```python
from build123d import *
from build123d.topology import SkipClean

# Parameters (mm, degrees)
BOSS_EXTRUDE1_DEPTH     = 8
FILLET2_R               = 2
SKETCH3_R               = 2.839661977
CUT_EXTRUDE1_DEPTH      = 8
SKETCH4_R               = 3.5
CUT_EXTRUDE2_DEPTH      = 8
CUT_EXTRUDE3_DEPTH      = 2.5
CUT_EXTRUDE3_DEPTH_BACK = 2.5
SKETCH5_R               = 32.5
SKETCH6_W               = 4.5
SKETCH6_H               = 19
CUT_EXTRUDE4_DEPTH      = 10
SKETCH7_R               = 1.75
CUT_EXTRUDE5_DEPTH      = 51
FILLET3_START           = -1
FILLET3_DEPTH           = 10
FILLET4_START           = -1
FILLET4_DEPTH           = 10
SKETCH9_W               = 5
SKETCH9_H               = 5
CUT_EXTRUDE6_DEPTH      = 51
SKETCH10_R              = 1.75
CUT_EXTRUDE7_DEPTH      = 24
FILLET5_DEPTH           = 1.5
FILLET5_START           = 6.5
FILLET5_2_DEPTH         = 1.5


with BuildPart() as part:
    # Sketch2 → Boss-Extrude1 (new body)
    with BuildSketch(Plane.XY):
        with BuildLine():
            Line((-102.95960155, 17.159933592), (-102.95960155, -17.159933592))
            add(Edge.make_bspline(
                [(-102.95960155, -17.159933592), (-76.189992309, -22.210205625), (-49.286425804, -24.488951052)],
                knots=[0, 0, 0, 0.320704871, 0.320704871, 0.320704871], degree=2))
            Line((-49.286425804, -24.488951052), (65.285160882, -24.488951052))
            Line((65.285160882, -24.488951052), (65.285160882, 24.488951052))
            Line((65.285160882, 24.488951052), (-49.286425804, 24.488951052))
            add(Edge.make_bspline(
                [(-102.95960155, 17.159933592), (-76.189992309, 22.210205625), (-49.286425804, 24.488951052)],
                knots=[0, 0, 0, 0.320704871, 0.320704871, 0.320704871], degree=2))
        make_face()
        with BuildLine():
            Line((-24.971677166, 17.771677006), (28.500163837, 17.771677006))
            Line((28.500163837, 17.771677006), (3.599814154, 4.650879462))
            ThreePointArc((3.599814154, 4.650879462), (1.764243335, 5), (-0.071327484, 4.650879462))
            Line((-0.071327484, 4.650879462), (-24.971677166, 17.771677006))
        make_face(mode=Mode.SUBTRACT)
        with BuildLine():
            Line((3.599814154, -4.650879462), (28.500163837, -17.771677006))
            Line((28.500163837, -17.771677006), (-24.971677166, -17.771677006))
            Line((-24.971677166, -17.771677006), (-0.071327484, -4.650879462))
            ThreePointArc((-0.071327484, -4.650879462), (1.764243335, -5), (3.599814154, -4.650879462))
        make_face(mode=Mode.SUBTRACT)
        with BuildLine():
            Line((-2.525196045, 2.569184657), (-26.859859934, 15.391904107))
            ThreePointArc((-26.859859934, 15.391904107), (-30.735756665, 0), (-26.859859934, -15.391904107))
            Line((-26.859859934, -15.391904107), (-2.525196045, -2.569184657))
            ThreePointArc((-2.525196045, -2.569184657), (-3.235756665, 0), (-2.525196045, 2.569184657))
        make_face(mode=Mode.SUBTRACT)
        with BuildLine():
            Line((6.053682716, -2.569184657), (30.388346604, -15.391904107))
            ThreePointArc((30.388346604, -15.391904107), (34.264243335, 0), (30.388346604, 15.391904107))
            Line((30.388346604, 15.391904107), (6.053682716, 2.569184657))
            ThreePointArc((6.053682716, 2.569184657), (6.764243335, 0), (6.053682716, -2.569184657))
        make_face(mode=Mode.SUBTRACT)
    extrude(amount=BOSS_EXTRUDE1_DEPTH)

    # Fillet2
    fillet2_edges = [part.edges().sort_by_distance(p)[0] for p in [
        (-24.971677166, 17.771677006, 4),
        (28.500163837, 17.771677006, 4),
        (-24.971677166, -17.771677006, 4),
        (28.500163837, -17.771677006, 4),
    ]]
    fillet(fillet2_edges, radius=FILLET2_R)

    # Sketch3 → Cut-Extrude1 (cut)
    with BuildSketch(Plane.XY.offset(8)):
        with Locations((53.859940094, 0)):
            Circle(SKETCH3_R)
    extrude(amount=-CUT_EXTRUDE1_DEPTH, mode=Mode.SUBTRACT)

    # Sketch4 → Cut-Extrude2 (cut)
    with BuildSketch(Plane.XY.offset(8)):
        with Locations((1.764243335, 0)):
            Circle(SKETCH4_R)
    extrude(amount=-CUT_EXTRUDE2_DEPTH, mode=Mode.SUBTRACT)

    # Sketch5 → Cut-Extrude3 (cut, two sides: drawn at the far end of the back side and taken through both)
    with SkipClean():  # the faces are left unmerged after this step: merging them gives an invalid solid
        with BuildSketch(Plane.XY.offset(4).offset(-CUT_EXTRUDE3_DEPTH_BACK)):
            with Locations((1.764243335, 0)):
                Circle(SKETCH5_R)
        extrude(amount=CUT_EXTRUDE3_DEPTH + CUT_EXTRUDE3_DEPTH_BACK, mode=Mode.SUBTRACT)

    # Sketch6 → Cut-Extrude4 (cut)
    with SkipClean():  # the faces are left unmerged after this step: merging them gives an invalid solid
        with BuildSketch(Plane.XY.offset(8)):
            with Locations((-52.644112073, 0)):
                Rectangle(SKETCH6_W, SKETCH6_H)
        extrude(amount=-CUT_EXTRUDE4_DEPTH, mode=Mode.SUBTRACT)

    # Sketch7 → Cut-Extrude5 (cut)
    with SkipClean():  # the faces are left unmerged after this step: merging them gives an invalid solid
        with BuildSketch(Plane(origin=(0, 24.488951052, 0), x_dir=(1, 0, 0), z_dir=(0, 1, 0))):
            with Locations(Location((45.285160882, -4, 0), (0, 0, 270))):
                Circle(SKETCH7_R)
        extrude(amount=-CUT_EXTRUDE5_DEPTH, mode=Mode.SUBTRACT)

    # Fillet3: read off the stored shape, not the designer's step
    # Fillet3 outline → Fillet3 (cut)
    with SkipClean():  # the faces are left unmerged after this step: merging them gives an invalid solid
        with BuildSketch(Plane.XY.offset(FILLET3_START)):
            with BuildLine():
                add(Edge.make_bspline(
                    [(-49.286425804, 24.488951052), (-55.269151656, 23.982211205), (-61.245253134, 23.338415518)],
                    knots=[0, 0, 0, 0.071317285, 0.071317285, 0.071317285], degree=2))
                ThreePointArc((-61.245253134, 23.338415518), (-50.549825889, 24.201110037), (-39.823523948, 24.488951052))
                Line((-39.823523948, 24.488951052), (-49.286425804, 24.488951052))
            make_face()
        extrude(amount=FILLET3_DEPTH, mode=Mode.SUBTRACT)

    # Fillet4: read off the stored shape, not the designer's step
    # Fillet4 outline → Fillet4 (cut)
    with SkipClean():  # the faces are left unmerged after this step: merging them gives an invalid solid
        with BuildSketch(Plane.XY.offset(FILLET4_START)):
            with BuildLine():
                Line((-49.286425804, -24.488951052), (-39.823523948, -24.488951052))
                ThreePointArc((-39.823523948, -24.488951052), (-50.549825889, -24.201110037), (-61.245253134, -23.338415518))
                add(Edge.make_bspline(
                    [(-61.245253134, -23.338415518), (-55.269151656, -23.982211205), (-49.286425804, -24.488951052)],
                    knots=[0.249387586, 0.249387586, 0.249387586, 0.320704871, 0.320704871, 0.320704871], degree=2))
            make_face()
        extrude(amount=FILLET4_DEPTH, mode=Mode.SUBTRACT)

    # Sketch9 → Cut-Extrude6 (cut)
    with SkipClean():  # the faces are left unmerged after this step: merging them gives an invalid solid
        with BuildSketch(Plane(origin=(0, 24.488951052, 0), x_dir=(1, 0, 0), z_dir=(0, 1, 0))):
            with Locations((-74.714839118, -4)):
                Rectangle(SKETCH9_W, SKETCH9_H)
        extrude(amount=-CUT_EXTRUDE6_DEPTH, mode=Mode.SUBTRACT)

    # Sketch10 → Cut-Extrude7 (cut)
    with SkipClean():  # the faces are left unmerged after this step: merging them gives an invalid solid
        with BuildSketch(Plane.ZY.offset(50.394112073)):
            with Locations((4, 0)):
                Circle(SKETCH10_R)
        extrude(amount=-CUT_EXTRUDE7_DEPTH, mode=Mode.SUBTRACT)

    # Fillet5: read off the stored shape, not the designer's step
    # Fillet5 outline → Fillet5 (add)
    with SkipClean():  # the faces are left unmerged after this step: merging them gives an invalid solid
        with BuildSketch(Plane.XY):
            with BuildLine():
                Line((30.388346604, 15.391904107), (25.603831674, 12.87078884))
                ThreePointArc((25.603831674, 12.87078884), (29.820861326, 13.077915151), (32.692963641, 9.983198898))
                ThreePointArc((32.692963641, 9.983198898), (31.663210239, 12.739771507), (30.388346604, 15.391904107))
            make_face()
            with BuildLine():
                ThreePointArc((30.388346604, -15.391904107), (31.663210239, -12.739771507), (32.692963641, -9.983198898))
                ThreePointArc((32.692963641, -9.983198898), (29.820861326, -13.077915151), (25.603831674, -12.87078884))
                Line((25.603831674, -12.87078884), (30.388346604, -15.391904107))
            make_face()
            with BuildLine():
                Line((-26.859859934, -15.391904107), (-22.075345003, -12.87078884))
                ThreePointArc((-22.075345003, -12.87078884), (-26.292374655, -13.077915151), (-29.164476971, -9.983198898))
                ThreePointArc((-29.164476971, -9.983198898), (-28.134723569, -12.739771507), (-26.859859934, -15.391904107))
            make_face()
            with BuildLine():
                ThreePointArc((-26.859859934, 15.391904107), (-28.134723569, 12.739771507), (-29.164476971, 9.983198898))
                ThreePointArc((-29.164476971, 9.983198898), (-26.292374655, 13.077915151), (-22.075345003, 12.87078884))
                Line((-22.075345003, 12.87078884), (-26.859859934, 15.391904107))
            make_face()
        extrude(amount=FILLET5_DEPTH)

    # Fillet5 2 outline → Fillet5 2 (add)
    with SkipClean():  # the faces are left unmerged after this step: merging them gives an invalid solid
        with BuildSketch(Plane.XY.offset(FILLET5_START)):
            with BuildLine():
                Line((30.388346604, 15.391904107), (25.603831674, 12.87078884))
                ThreePointArc((25.603831674, 12.87078884), (29.820861326, 13.077915151), (32.692963641, 9.983198898))
                ThreePointArc((32.692963641, 9.983198898), (31.663210239, 12.739771507), (30.388346604, 15.391904107))
            make_face()
            with BuildLine():
                ThreePointArc((30.388346604, -15.391904107), (31.663210239, -12.739771507), (32.692963641, -9.983198898))
                ThreePointArc((32.692963641, -9.983198898), (29.820861326, -13.077915151), (25.603831674, -12.87078884))
                Line((25.603831674, -12.87078884), (30.388346604, -15.391904107))
            make_face()
            with BuildLine():
                Line((-26.859859934, -15.391904107), (-22.075345003, -12.87078884))
                ThreePointArc((-22.075345003, -12.87078884), (-26.292374655, -13.077915151), (-29.164476971, -9.983198898))
                ThreePointArc((-29.164476971, -9.983198898), (-28.134723569, -12.739771507), (-26.859859934, -15.391904107))
            make_face()
            with BuildLine():
                ThreePointArc((-26.859859934, 15.391904107), (-28.134723569, 12.739771507), (-29.164476971, 9.983198898))
                ThreePointArc((-29.164476971, 9.983198898), (-26.292374655, 13.077915151), (-22.075345003, 12.87078884))
                Line((-22.075345003, 12.87078884), (-26.859859934, 15.391904107))
            make_face()
        extrude(amount=FILLET5_2_DEPTH)


solid = part.part
```
Geometry: final body of the model. Coordinates: model frame, mm. A direction names the side the tool comes from. Round coordinates to 2 decimals unless told otherwise and drop trailing zeros. Write item = value, one per line. Start each with the question number.
Q1. Pull-direction query (X, two-part tool) for faces 1 (the cylindrical face through (30, 13, 1)), 2 (the flat face through (-102.96, 0, 4)); classes: +X half, -X half, draft (parallel to the pull), parting line (faces both ways), or undercut.
Q2. Access query for faces 3 (the flat face through (-75, 0, 1.5)), 4 (the cylindrical face through (-50.7, 24.193, 3.944)), 5 (the cylindrical face through (-40.68, 0.08, 2.25)), 6 (the flat face through (-12.437, -7.792, 0.74)). Directions: +Z, -Z, +X, -X, +Y, -Y. A direction counts if a zero-diameter tool reaches every point of the face in a straight line with its end or side. Return the directions, or none.
Q3. Cut plane A-A on z = 4. Give the number of separate pieces and of enclosed holes in the cut face, and give its area (3 significant figures).
Q4. Pin query (flat end, axial travel): pin 1 (2 mm diameter, centred on x = -52.5, z = 3.5, fed in from +Y). Return the tip coordinate at first contact, or that it passes through.
Q5. Ray query, line 1 (X direction, y = -10, z = 1.75); line 2 (Y direction, x = -36, z = 4); line 3 (X direction, y = -5.5, z = 5). Return the intervals inside material, ascending. Write a range as from..to.
Outcome:
q1.face_1 = undercut
q1.face_2 = -X half
q2.face_3 = +Y, -Y
q2.face_4 = +Z, -Z, -X, +Y
q2.face_5 = none
q2.face_6 = +Z, -Z
q3.separate_pieces = 4
q3.enclosed_holes = 1
q3.area = 4,480 mm^2
q4.pin_1 = 24.15
q5.line_1 = -102.96..-77.21, -72.21..-29.16, 32.69..65.29
q5.line_2 = -24.49..-1.75, 1.75..24.49
q5.line_3 = -102.96..-77.21, -72.21..-54.89, -50.39..-30.27, 33.8..43.85, 46.72..65.29
